Geometry: final body of the model. Coordinates: model frame, mm. Give positions to 0.01 mm unless a question says otherwise; leave off trailing zeros. Order: outer loops, then holes, each group sorted by start corner. A loop starts at its lowest first (then second) coordinate and runs counter-clockwise, first axis right, second up. Notation, with made-up numbers: (-39.75, 1) - (-21.75, 1) arc R29 cw to (-21.75, 38) - close; hole circle Ø6 at (72.5, 3.25). An arc over 180 degrees is marked (long way). One line per item, written item: value.
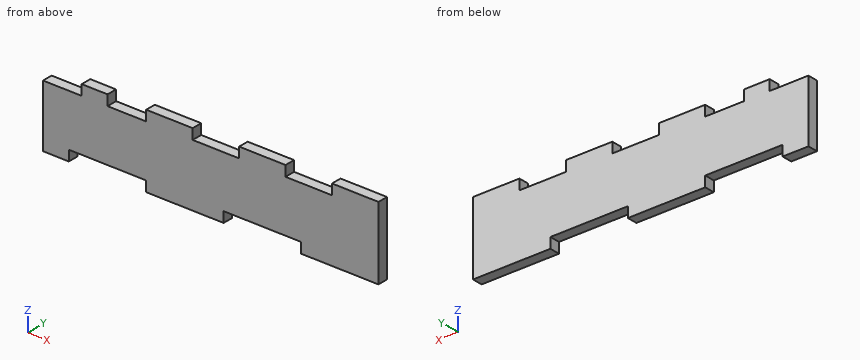
```python
from build123d import *

# Parameters (mm, degrees)
BOSS_EXTRUDE1_DEPTH = 2


with BuildPart() as part:
    # Sketch1 → Boss-Extrude1 (new, symmetric)
    with BuildSketch(Plane(origin=(0, 0, 0), x_dir=(1, 0, 0), z_dir=(0, 1, 0))):
        Polygon((-65, -10), (-50, -10), (-50, -14), (-40, -14), (-40, -10), (-25, -10), (-25, -14), (-7, -14), (-7, -10), (11, -10), (11, -14), (29, -14), (29, -10), (47, -10), (47, -14), (65, -14), (65, -10), (65, 10), (65, 14), (35, 14), (35, 10), (5, 10), (5, 14), (-25, 14), (-25, 10), (-55, 10), (-55, 14), (-65, 14), (-65, 10), align=None)
    extrude(amount=BOSS_EXTRUDE1_DEPTH, both=True)


solid = part.part
```
1) Section B-B, the plane x = -34. Return loops of the section in (y, z).
Answers below:
outline: (-2, -10) - (2, -10) - (2, 10) - (-2, 10) - close
2) Section A-A, the plane y = 1. Return loops of the section in (x, z), then the cut area to 3 significant figures.
Answers below:
outline: (-65, -14) - (-55, -14) - (-55, -10) - (-25, -10) - (-25, -14) - (5, -14) - (5, -10) - (35, -10) - (35, -14) - (65, -14) - (65, 14) - (47, 14) - (47, 10) - (29, 10) - (29, 14) - (11, 14) - (11, 10) - (-7, 10) - (-7, 14) - (-25, 14) - (-25, 10) - (-40, 10) - (-40, 14) - (-50, 14) - (-50, 10) - (-65, 10) - close
area: 3,140 mm^2
3) Section C-C, the plane x = 41.5. Return loops of the section in (y, z).
Answers below:
outline: (-2, -14) - (2, -14) - (2, 10) - (-2, 10) - close
4) Material intervals for line 1 along X through (y, z) = (-1.65, 10.5); line 2 along X through (y, z) = (-0.1, -11.5); line 3 along Z through (x, y) = (-40.5, 0.65), sorted ascending.
Answers below:
line 1: -50 to -40, -25 to -7, 11 to 29, 47 to 65
line 2: -65 to -55, -25 to 5, 35 to 65
line 3: -10 to 14
